Work out the finished part from the listing and answer in its coordinate system (mm). Face numbers are marked on the shaded views. A direction names the side the tool comes from. Round coordinates to 2 decimals unless told otherwise and drop trailing zeros. Write each loop counter-clockwise with the first axis right and the second up, starting at its lowest first coordinate (ties: lowest second). Pieces come first, ordered by that corner, then holes. Notation, with made-up numbers: M 9.5,10.5 L 59.5,10.5 A26 cw 59.5,25.5 Z; hole C -1.75,8 d5. An arc over 180 degrees is marked long. One line per item, written item: value. Start each with the question number.
Q1. Find section C-C (z = -10.5). Write down the section's boundary in (x, y).
Q2. Find section D-D (y = 3.75). Write down the section's boundary in (x, z).
Q3. Find section B-B (z = -5.5). Write down the section's boundary in (x, y), and give its area (3 significant figures).
Q4. The mould has two halves that part along X. Classify the marked faces 1, 2 and 3: released by +X, released by -X, zero draft, split by the parting line, or undercut.
Q5. A tool of negligible diameter and unlimited length cuts with its end or side. For the marked faces 4 and 5, from which of +Z, -Z, +X, -X, +Y, -Y can it reach the whole face along a straight path? Write none if from no direction.
Q6. Consider probe 1 along Z at (x, y) = (-24, 4.05); probe 2 along X at (y, z) = (13.55, 15.5); probe 3 along X at (y, z) = (2.7, -16). Determine where each line is inside the solid, lowest interval first.
Q7. Find section A-A (x = 24). Write down the section's boundary in (y, z).
Q8. Given pin 1 Ø5 at (x, z) = (16, -5.5) entering from -Y; pin 2 Ø1.8 at (x, z) = (-14, 15.5) entering from +Y; pin 3 Ø10 at (x, y) = (12, 9.5) entering from -Z; pin 4 Ø3.5 at (x, z) = (-24, -5.5) entering from +Y, each flat-ended and moving along its own axis, determine where each tip first touches the part or whether it passes through.
from build123d import *

# Parameters (mm, degrees)
BOSS_EXTRUDE1_DEPTH = 5
SKETCH2_R           = 1.5
CUT_EXTRUDE1_DEPTH  = 6
SKETCH3_W           = 54
SKETCH3_H           = 10
BOSS_EXTRUDE2_DEPTH = 13
SKETCH4_R           = 1
CUT_EXTRUDE2_DEPTH  = 6


with BuildPart() as part:
    # Sketch1 → Boss-Extrude1 (new body)
    with BuildSketch(Plane(origin=(0, 0, 0), x_dir=(1, 0, 0), z_dir=(0, 1, 0))):
        Polygon((-20, 20.75), (-20, 0.75), (20, 0.75), (20, 20.75), (27, 20.75), (27, -20.75), (-27, -20.75), (-27, 20.75), align=None)
    extrude(amount=BOSS_EXTRUDE1_DEPTH)

    # Sketch2 → Cut-Extrude1 (cut, through all)
    with BuildSketch(Plane(origin=(0, 5, 0), x_dir=(1, 0, 0), z_dir=(0, 1, 0))):
        with Locations((-24, 16)):
            Circle(SKETCH2_R)
        with Locations((-24, 5.5)):
            Circle(SKETCH2_R)
        with Locations((24, 16)):
            Circle(SKETCH2_R)
        with Locations((24, 5.5)):
            Circle(SKETCH2_R)
    extrude(amount=-CUT_EXTRUDE1_DEPTH, mode=Mode.SUBTRACT)

    # Sketch3 → Boss-Extrude2 (add)
    with BuildSketch(Plane(origin=(0, 5, 0), x_dir=(1, 0, 0), z_dir=(0, 1, 0))):
        with Locations((0, -15.75)):
            Rectangle(SKETCH3_W, SKETCH3_H)
    extrude(amount=BOSS_EXTRUDE2_DEPTH)

    # Sketch4 → Cut-Extrude2 (cut)
    with BuildSketch(Plane(origin=(0, 18, 0), x_dir=(1, 0, 0), z_dir=(0, 1, 0))):
        with Locations((-14, -15.5)):
            Circle(SKETCH4_R)
        with Locations((9.5, -15.5)):
            Circle(SKETCH4_R)
    extrude(amount=-CUT_EXTRUDE2_DEPTH, mode=Mode.SUBTRACT)


solid = part.part
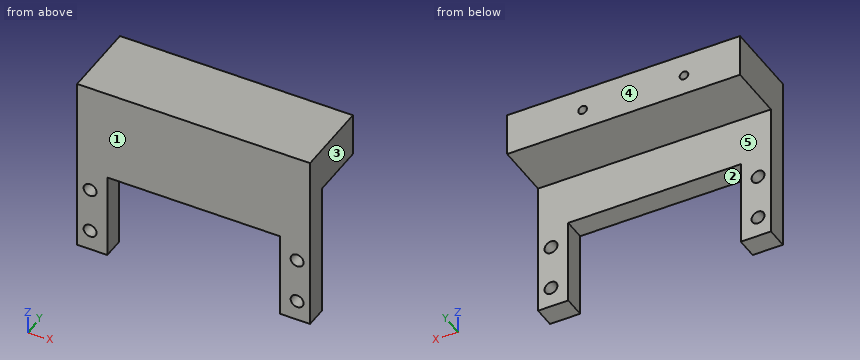
The answers:
1. outline: M -27,0 L -20,0 L -20,5 L -27,5 Z; M 20,0 L 27,0 L 27,5 L 20,5 Z
2. outline: M -27,-20.75 L -20,-20.75 L -20,-0.75 L 20,-0.75 L 20,-20.75 L 27,-20.75 L 27,20.75 L -27,20.75 Z; hole C -24,-16 d3; hole C -24,-5.5 d3; hole C 24,-16 d3; hole C 24,-5.5 d3
3. outline: M -27,0 L -25.5,0 L -25.5,5 L -27,5 Z; M -22.5,0 L -20,0 L -20,5 L -22.5,5 Z; M 20,0 L 22.5,0 L 22.5,5 L 20,5 Z; M 25.5,0 L 27,0 L 27,5 L 25.5,5 Z
3. area: 40.0 mm2
4. face 1: zero draft
4. face 2: undercut
4. face 3: released by +X
5. face 4: +Z, -Z, +X, -X, +Y
5. face 5: -Z, +X, -X, +Y
6. probe 1: -20.75 to -17.5, -14.5 to -7, -4 to 20.75
6. probe 2: -27 to -15, -13 to 8.5, 10.5 to 27
6. probe 3: -27 to -25.5, -22.5 to -20, 20 to 22.5, 25.5 to 27
7. outline: M 0,-20.75 L 5,-20.75 L 5,-17.5 L 0,-17.5 Z; M 0,-14.5 L 5,-14.5 L 5,-7 L 0,-7 Z; M 0,-4 L 5,-4 L 5,10.75 L 18,10.75 L 18,20.75 L 0,20.75 Z
8. pin 1: through
8. pin 2: y = 12
8. pin 3: z = -0.75
8. pin 4: y = 5
